Part model, mm, in its own coordinate system. Coordinates: 2 decimals unless noted, no trailing zeros. Write each loop counter-clockwise with the first axis right and the second up, starting at its lowest first coordinate (ties: lowest second). Pieces come first, ordered by that corner, then holes. Notation, with made-up numbers: (-7.75, -22.5) -> (19.25, -22.5) arc R35 ccw to (19.25, 11.5) -> close; hole circle Ø6 at (26.5, -1.5). An arc over 180 degrees is marked (long way). Write item = value, one per line. Start each with the question number.
Q1. Probe line 1 (Z direction, x = 353.5, y = -2.35); line 2 (X direction, y = -0.45, z = 173); line 3 (Z direction, x = 358, y = -0.8). List the from-to ranges inside material, lowest first.
Q2. Pin check, flat tips, straight feed: P1, Ø1.7, axis at x = 212.5, y = -2.5, coming from the -Z side; P2, Ø8, axis at x = 191.5, z = 202.5, coming from the +Y side; P3, Ø1.5, axis at x = 382.5, y = -1.5, coming from the -Z side; P4, Ø1.7, axis at x = 385, y = -2, coming from the +Z side. Stop position of each tip, or through.
Q3. Band-saw the part on D-D, the plane x = 253. List the corners of the cut face in (y, z).
Q4. Band-saw the part on A-A, the plane x = 193. List the corners of the cut face in (y, z).
Q5. Band-saw the part on C-C, the plane z = 181. List the corners of the cut face in (x, y), plus the area to 3 significant figures.
Q6. Band-saw the part on B-B, the plane z = 159. List the corners of the cut face in (x, y), plus the area to 3 significant figures.
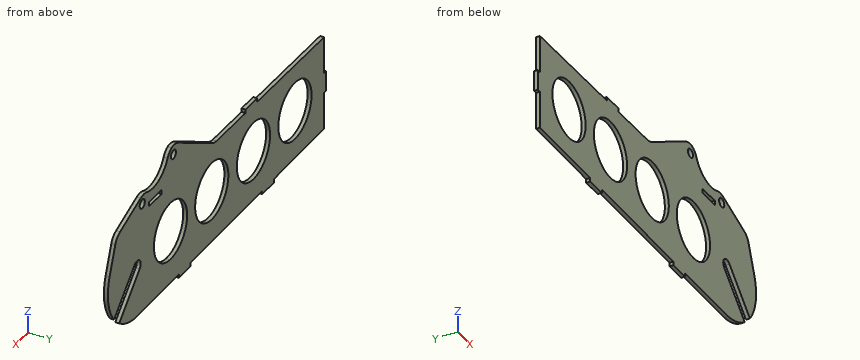
from build123d import *

# Parameters (mm, degrees)
F0_R     = 25.4
F0_W     = 19.05
F0_H     = 3.81
F0_R_2   = 3.81
F0_R_3   = 3.937
F1_DEPTH = 3.429


# Not quite as in the source:
# - ends of sketch curves that miss each other by under 0.0002 mm in the source are joined


with BuildPart() as f1:
    # F0 (on Front) → F1 (new body)
    with BuildSketch(Plane.XZ):
        with BuildLine():
            Line((122.9326218, 166.8279366), (126.1076218, 166.8279366))
            Line((126.1076218, 166.8279366), (126.1076218, 134.4429366))
            Line((126.1076218, 134.4429366), (202.8156218, 132.7586372))
            Line((202.8156218, 132.7586372), (202.8156218, 129.4566372))
            Line((202.8156218, 129.4566372), (220.5956218, 129.4566372))
            Line((220.5956218, 129.4566372), (220.5956218, 132.3682392))
            Line((220.5956218, 132.3682392), (330.0696218, 129.9644848))
            Line((330.0696218, 129.9644848), (330.0696218, 126.6616974))
            Line((330.0696218, 126.6616974), (347.7771302, 126.2728742))
            Line((347.7771302, 126.2728742), (347.8496218, 129.5740868))
            Line((347.8496218, 129.5740868), (413.8162158, 128.1256518))
            ThreePointArc((413.8162158, 128.1256518), (427.2355191442, 130.7449674015), (439.2238892088, 137.3189752107))
            Line((439.2238892088, 137.3189752107), (407.9287752, 168.61409))
            ThreePointArc((407.9287752, 168.61409), (407.928759747, 176.471798653), (415.786483853, 176.471798653))
            Line((415.786483853, 176.471798653), (447.1136092, 145.1446932))
            ThreePointArc((447.1136092, 145.1446932), (456.0111791953, 165.5693177048), (453.8809524214, 187.7457494791))
            Line((453.8809524214, 187.7457494791), (445.1949186, 211.6104734))
            ThreePointArc((445.1949186, 211.6104734), (442.3538053066, 216.1328975514), (437.9046056469, 219.0873571921))
            Line((437.9046056469, 219.0873571921), (406.246711, 231.5244036))
            ThreePointArc((406.246711, 231.5244036), (401.6620386638, 232.4037156495), (397.069381607, 231.5671130188))
            ThreePointArc((397.069381607, 231.5671130188), (378.7147395647, 231.6525545857), (365.2100276158, 244.0832755023))
            ThreePointArc((365.2100276158, 244.0832755023), (362.7212006534, 247.5307318984), (359.2339287197, 249.9634606203))
            ThreePointArc((359.2339287197, 249.9634606203), (354.0189561213, 250.4862087964), (349.0369734787, 248.858627921))
            Line((349.0369734787, 248.858627921), (296.7910244, 218.6944318))
            ThreePointArc((296.7910244, 218.6944318), (293.728030578, 217.4256797597), (290.4410244, 216.9929366))
            Line((290.4410244, 216.9929366), (246.1226218, 216.9929366))
            Line((246.1226218, 216.9929366), (246.1226218, 220.1679366))
            Line((246.1226218, 220.1679366), (228.3426218, 220.1679366))
            Line((228.3426218, 220.1679366), (228.3426218, 216.9929366))
            Line((228.3426218, 216.9929366), (126.1076218, 216.9929366))
            Line((126.1076218, 216.9929366), (126.1076218, 184.6079366))
            Line((126.1076218, 184.6079366), (122.9326218, 184.6079366))
            Line((122.9326218, 184.6079366), (122.9326218, 166.8279366))
        make_face()
        with Locations((170.5510686, 175.9319824)):
            Circle(F0_R, mode=Mode.SUBTRACT)
        with Locations((233.9839364, 175.9319824)):
            Circle(F0_R, mode=Mode.SUBTRACT)
        with Locations((297.721782, 175.9319824)):
            Circle(F0_R, mode=Mode.SUBTRACT)
        with Locations((360.7561746, 175.9319824)):
            Circle(F0_R, mode=Mode.SUBTRACT)
        with Locations((383.9176218, 218.8979366)):
            Rectangle(F0_W, F0_H, mode=Mode.SUBTRACT)
        with Locations((356.2316218, 242.3929366)):
            Circle(F0_R_2, mode=Mode.SUBTRACT)
        with Locations((403.935946, 224.9304366)):
            Circle(F0_R_3, mode=Mode.SUBTRACT)
    extrude(amount=F1_DEPTH)


solid = f1.part
Ans:
q1.line_1 = 129.45 to 151.59, 200.27 to 239.74, 245.05 to 250.42
q1.line_2 = 122.93 to 145.32, 195.78 to 208.75, 259.21 to 272.49, 322.95 to 335.53, 385.99 to 406.32, 419.26 to 456.56
q1.line_3 = 129.35 to 150.68, 201.18 to 239.02, 245.77 to 250.29
q2.P1 = 129.46
q2.P2 = 0
q2.P3 = 128.8
q2.P4 = 230.19
q3.outline = (-3.43, 131.66) -> (0, 131.66) -> (0, 159.09) -> (-3.43, 159.09) -> close; (-3.43, 192.77) -> (0, 192.77) -> (0, 216.99) -> (-3.43, 216.99) -> close
q4.outline = (-3.43, 132.97) -> (0, 132.97) -> (0, 164.05) -> (-3.43, 164.05) -> close; (-3.43, 187.81) -> (0, 187.81) -> (0, 216.99) -> (-3.43, 216.99) -> close
q5.outline = (122.93, -3.43) -> (145.66, -3.43) -> (145.66, 0) -> (122.93, 0) -> close; (195.44, -3.43) -> (209.09, -3.43) -> (209.09, 0) -> (195.44, 0) -> close; (258.87, -3.43) -> (272.83, -3.43) -> (272.83, 0) -> (258.87, 0) -> close; (322.61, -3.43) -> (335.87, -3.43) -> (335.87, 0) -> (322.61, 0) -> close; (385.65, -3.43) -> (455.75, -3.43) -> (455.75, 0) -> (385.65, 0) -> close
q5.area = 458 mm2
q6.outline = (126.11, -3.43) -> (151.62, -3.43) -> (151.62, 0) -> (126.11, 0) -> close; (189.48, -3.43) -> (215.05, -3.43) -> (215.05, 0) -> (189.48, 0) -> close; (252.92, -3.43) -> (278.79, -3.43) -> (278.79, 0) -> (252.92, 0) -> close; (316.66, -3.43) -> (341.82, -3.43) -> (341.82, 0) -> (316.66, 0) -> close; (379.69, -3.43) -> (417.54, -3.43) -> (417.54, 0) -> (379.69, 0) -> close; (433.26, -3.43) -> (454.45, -3.43) -> (454.45, 0) -> (433.26, 0) -> close
q6.area = 553 mm2
